```python
from build123d import *

# Parameters (mm, degrees)
SKETCH_1_W                  = 240
SKETCH_1_H                  = 150
EXTRUDE_1_DEPTH             = 16
SKETCH_2_R                  = 10.728301902
CUT_EXTRUDE_1_DEPTH         = 284.471338939
PATTERN_LINEAR_1_COUNT      = 2
PATTERN_LINEAR_1_PITCH      = 170
PATTERN_LINEAR_1_COUNT_DIR2 = 2
PATTERN_LINEAR_1_PITCH_DIR2 = 80
SKETCH_3_W                  = 6
SKETCH_3_H                  = 150
EXTRUDE_2_DEPTH             = 80
CUT_EXTRUDE_2_DEPTH         = 243.777676074
SKETCH_7_W                  = 240
SKETCH_7_H                  = 16
EXTRUDE_3_DEPTH             = 144
CUT_EXTRUDE_4_DEPTH         = 301.14829668
CUT_EXTRUDE_5_DEPTH         = 301.14829668
SKETCH_15_R                 = 19.766227273
CUT_EXTRUDE_6_DEPTH         = 301.14829668


with BuildPart() as part:
    # 草图1 → 凸台-拉伸1 (new body)
    with BuildSketch(Plane(origin=(0, 0, 0), x_dir=(1, 0, 0), z_dir=(0, 1, 0))):
        with Locations((120, 75)):
            Rectangle(SKETCH_1_W, SKETCH_1_H)
    extrude(amount=EXTRUDE_1_DEPTH)

    # 草图2 → 切除-拉伸1 (cut, through all)
    with BuildSketch(Plane(origin=(0, 16, 0), x_dir=(1, 0, 0), z_dir=(0, 1, 0))):
        with Locations(Location((35, 35, 0), (0, 0, 270))):
            Circle(SKETCH_2_R)
    cut_extrude_1 = extrude(amount=-CUT_EXTRUDE_1_DEPTH, mode=Mode.SUBTRACT)

    # 阵列(线性)1: Cut-Extrude 1 2 × 2
    with Locations(*[(i * PATTERN_LINEAR_1_PITCH, 0, -j * PATTERN_LINEAR_1_PITCH_DIR2) for i in range(PATTERN_LINEAR_1_COUNT) for j in range(PATTERN_LINEAR_1_COUNT_DIR2) if (i, j) != (0, 0)]):
        add(cut_extrude_1, mode=Mode.SUBTRACT)

    # 草图3 → 凸台-拉伸2 (add)
    with BuildSketch(Plane(origin=(0, 16, 0), x_dir=(1, 0, 0), z_dir=(0, 1, 0))):
        with Locations((168, 75)):
            Rectangle(SKETCH_3_W, SKETCH_3_H)
    extrude(amount=EXTRUDE_2_DEPTH)

    # 草图4 → 切除-拉伸2 (cut, through all)
    with BuildSketch(Plane.ZY.offset(-165)):
        Polygon((0, 96), (-47, 96), (0, 36), align=None)
        Polygon((-150, 96), (-103, 96), (-150, 36), align=None)
    extrude(amount=-CUT_EXTRUDE_2_DEPTH, mode=Mode.SUBTRACT)

    # 草图7 → 凸台-拉伸3 (add)
    with BuildSketch(Plane(origin=(0, 16, 0), x_dir=(1, 0, 0), z_dir=(0, 1, 0))):
        with Locations((120, 75)):
            Rectangle(SKETCH_7_W, SKETCH_7_H)
    extrude(amount=EXTRUDE_3_DEPTH)

    # 草图12 → 切除-拉伸4 (cut, through all)
    with BuildSketch(Plane.XY.offset(-67)):
        with BuildLine():
            Line((32.874495942, 118.348754348), (0, 16))
            Line((0, 16), (0, 160))
            Line((0, 160), (90, 160))
            ThreePointArc((90, 160), (54.651204129, 148.481570008), (32.874495942, 118.348754348))
        make_face()
    extrude(amount=-CUT_EXTRUDE_4_DEPTH, mode=Mode.SUBTRACT)

    # 草图14 → 切除-拉伸5 (cut, through all)
    with BuildSketch(Plane.XY.offset(-67)):
        with BuildLine():
            Line((132.198608493, 142.652988656), (240, 36))
            Line((240, 36), (240, 160))
            Line((240, 160), (90, 160))
            ThreePointArc((90, 160), (112.812504035, 155.494050669), (132.198608493, 142.652988656))
        make_face()
    extrude(amount=-CUT_EXTRUDE_5_DEPTH, mode=Mode.SUBTRACT)

    # 草图15 → 切除-拉伸6 (cut, through all)
    with BuildSketch(Plane.XY.offset(-67)):
        with Locations((90, 100)):
            Circle(SKETCH_15_R)
    extrude(amount=-CUT_EXTRUDE_6_DEPTH, mode=Mode.SUBTRACT)


solid = part.part
```
Build history of the part. All positions in model axes, mm. A direction names the side the tool comes from. Round coordinates to 2 decimals unless told otherwise and drop trailing zeros. Loops run counter-clockwise (first coordinate to the right, second up) from the corner with the lowest first, then second, coordinate; pieces in that order, holes last.
Item 1: Two-plate mould, pull along X, no slides. Class faces 1 (the face through (167.96, 66.42, -23.83)), 2 (the face through (195.48, 8.11, -110.05)), 3 (the face through (171, 47, -109)): released by +X, released by -X, zero draft, split by the parting line, or undercut.
Item 2: Saw through at B-B (y = 100). List the corners of the cut face in (x, z), then the cut area to 3 significant figures.
Item 3: Saw through at C-C (z = -41.5). List the corners of the cut face in (x, y).
Item 4: Saw through at A-A (z = -72). List the corners of the cut face in (x, y).
Item 5: Pin check, flat tips, straight feed: P1, Ø12, axis at x = 91, z = -91.5, coming from the +Y side; P2, Ø4, axis at x = 29.5, y = 65.5, coming from the +Z side; P3, Ø6.5, axis at x = 169, z = -55, coming from the +Y side. Stop position of each tip, or through.
Item 6: Drill centre lines: line 1 along X through (y, z) = (10.75, -115); line 2 along Y through (x, z) = (90, -74.25); line 3 along Y through (x, z) = (142, -51). Where is each one in solid material? Low to high.
Item 7: Saw through at D-D (z = -88). List the corners of the cut face in (x, y).
Item 8: Which spindle directions (+Z, -Z, +X, -X, +Y, -Y) get a long thin tool onto all of the face, cutting with end or side? Do faces 4 (the face through (197, 16, -124)), 5 (the face through (197, 16, -27)), 6 (the face through (165, 47, -40)). Say none if no direction does.
Worked answers:
1. face 1: zero draft
1. face 2: undercut
1. face 3: released by +X
2. outline: (26.98, -83) - (70.23, -83) - (70.23, -67) - (26.98, -67) - close; (109.77, -83) - (175.31, -83) - (175.31, -67) - (109.77, -67) - close
2. area: 1,740 mm2
3. outline: (0, 0) - (26.46, 0) - (26.46, 16) - (0, 16) - close; (43.54, 0) - (196.46, 0) - (196.46, 16) - (171, 16) - (171, 88.98) - (165, 88.98) - (165, 16) - (43.54, 16) - close; (213.54, 0) - (240, 0) - (240, 16) - (213.54, 16) - close
4. outline: (0, 0) - (240, 0) - (240, 36) - (132.2, 142.65) arc R60 ccw to (32.87, 118.35) - (0, 16) - close; hole circle Ø39.53 at (90, 100)
5. P1: stops at y = 16
5. P2: stops at z = -67
5. P3: stops at y = 96
6. line 1: x = 0 to 24.27, 45.73 to 194.27, 215.73 to 240
6. line 2: y = 0 to 80.23, 119.77 to 160
6. line 3: y = 0 to 16
7. outline: (0, 0) - (240, 0) - (240, 16) - (171, 16) - (171, 96) - (165, 96) - (165, 16) - (0, 16) - close
8. face 4: -Z, +X, +Y
8. face 5: +Z, +X, +Y
8. face 6: +Z, -X, +Y
